Can you work these out from the model? Positions are in its coordinate system, mm. A direction names the side the tool comes from. Round coordinates to 2 decimals unless told otherwise and drop trailing zeros. Loops run counter-clockwise (first coordinate to the right, second up) from the corner with the lowest first, then second, coordinate; pieces in that order, holes last.
from build123d import *

# Parameters (mm, degrees)
F0_R     = 5
F1_DEPTH = 7.75
F2_R     = 1.25
F3_DEPTH = 25
F4_R     = 5
F5_DEPTH = 7.75
F6_R     = 1.25
F7_DEPTH = 25


with BuildPart() as f1:
    # F0 (on Front) → F1 (new body, symmetric)
    with BuildSketch(Plane.XZ):
        Circle(F0_R)
    extrude(amount=F1_DEPTH, both=True)

    # F2 (on face) → F3 (cut)
    with BuildSketch(Plane.XZ.offset(7.75)):
        Circle(F2_R)
    extrude(amount=-F3_DEPTH, mode=Mode.SUBTRACT)

    # F4 (on Right) → F5 (join, symmetric)
    with BuildSketch(Plane.YZ):
        Circle(F4_R)
    extrude(amount=F5_DEPTH, both=True)

    # F6 (on face) → F7 (cut)
    with BuildSketch(Plane.YZ.offset(7.75)):
        Circle(F6_R)
    extrude(amount=-F7_DEPTH, mode=Mode.SUBTRACT)


solid = f1.part
(1) If we section it at A-A, the plane z = 0: List the corners of the cut face in (x, y) for me.
Worked answers:
outline: (-7.75, -5) - (-5, -5) - (-5, -7.75) - (-1.25, -7.75) - (-1.25, -5) - (1.25, -5) - (1.25, -7.75) - (5, -7.75) - (5, -5) - (7.75, -5) - (7.75, -1.25) - (-7.75, -1.25) - close; (-7.75, 1.25) - (7.75, 1.25) - (7.75, 5) - (5, 5) - (5, 7.75) - (1.25, 7.75) - (1.25, 5) - (-1.25, 5) - (-1.25, 7.75) - (-5, 7.75) - (-5, 5) - (-7.75, 5) - close
(2) Will this pin go through, and if not, where does the flat tip stop? P1, Ø1.5, axis at x = 0, z = 0, coming from the -Y side.
Worked answers:
P1: stops at y = -5
(3) If I drill on line 1 (Z direction, x = 2, y = 0); line 2 (Y direction, x = 0, z = 0.75), over which ranges is the centre line in solid material (lowest first)?
Worked answers:
line 1: z = -5 to -1.25, 1.25 to 5
line 2: y = -4.94 to -1, 1 to 4.94
(4) If we section it at D-D, the plane x = 0.25: List the corners of the cut face in (y, z) for me.
Worked answers:
outline: (-7.75, -4.99) - (-0.25, -4.99) arc R5 ccw to (0.25, -4.99) - (7.75, -4.99) - (7.75, -1.22) - (4.85, -1.22) arc R5 ccw to (4.85, 1.22) - (7.75, 1.22) - (7.75, 4.99) - (0.25, 4.99) arc R5 ccw to (-0.25, 4.99) - (-7.75, 4.99) - (-7.75, 1.22) - (-4.85, 1.22) arc R5 ccw to (-4.85, -1.22) - (-7.75, -1.22) - close; hole circle Ø2.5 at (0, 0)
(5) If we mould it in two halves opening along X, with no side actions, what happens to faces 5 (the cylindrical face through (4.77, -5.65, 1.5)), 6 (the cylindrical face through (0, -5, 0)), 7 (the flat face through (1, -7.75, -1))? For each: released by +X, released by -X, zero draft, split by the parting line, or undercut.
Worked answers:
face 5: split by the parting line
face 6: undercut
face 7: zero draft
(6) If we section it at B-B, the plane y = 0.5: List the corners of the cut face in (x, z) for me, then the cut area to 3 significant figures.
Worked answers:
outline: (-7.75, -4.97) - (-0.5, -4.97) arc R5 ccw to (0.5, -4.97) - (7.75, -4.97) - (7.75, -1.15) - (-7.75, -1.15) - close; (-7.75, 1.15) - (7.75, 1.15) - (7.75, 4.97) - (0.5, 4.97) arc R5 ccw to (-0.5, 4.97) - (-7.75, 4.97) - close
area: 119 mm2
(7) If we section it at C-C, the plane z = -3: List the corners of the cut face in (x, y) for me.
Worked answers:
outline: (-7.75, -4) - (-4, -4) - (-4, -7.75) - (4, -7.75) - (4, -4) - (7.75, -4) - (7.75, 4) - (4, 4) - (4, 7.75) - (-4, 7.75) - (-4, 4) - (-7.75, 4) - close
(8) For faces 1 (the cylindrical face through (5.65, 4.77, 1.5)), 2 (the cylindrical face through (-0.27, -6.32, -1.22)), 3 (the cylindrical face through (-5.543, -0.651, 4.957)), 4 (the cylindrical face through (-0.27, 6.28, -1.22)), which set-ups out of +Z, -Z, +X, -X, +Y, -Y let a thin tool reach every point of the face, with its end or its side?
Worked answers:
face 1: +X
face 2: -Y
face 3: -X
face 4: +Y
